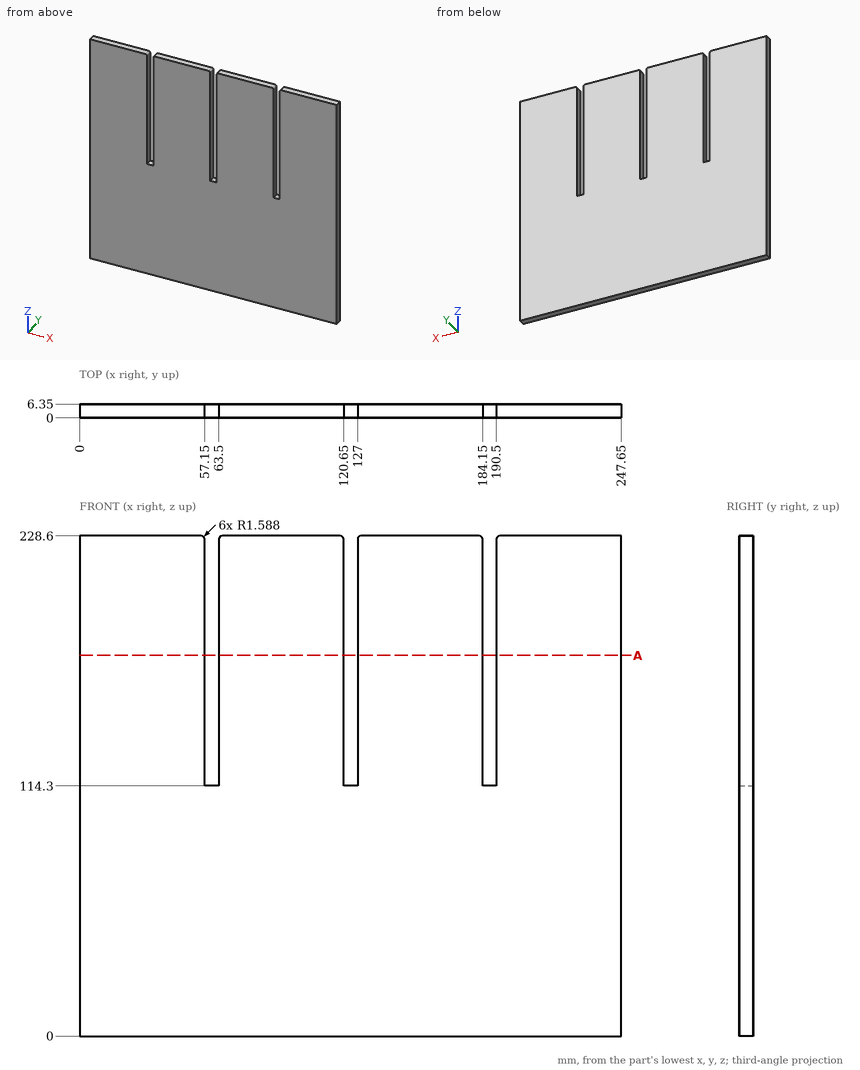
Can you work these out from the drawing? Everything is in mm from the part's minimum corner. Round coordinates to 2 decimals unless told otherwise and drop trailing zeros. Order: outer loops, then holes, each group sorted by start corner. A loop starts at its lowest first (then second) coordinate and runs counter-clockwise, first axis right, second up. Notation, with made-up numbers: (56, 7.5) -> (63, 7.5) arc R19 cw to (63, 27.5) -> close; hole circle Ø6 at (-6.5, 47.25). An arc over 180 degrees is marked (long way). Use CSV: the item, a comma, the result in double quotes.
1. I'm going to push flat-ended pins straight in: P1, Ø1.9, axis at x = 123.5, y = 3.5, coming from the +Z side; P2, Ø3, axis at y = 3, z = 192.5, coming from the -X side. Where does each tip first touch, or does it pass through?
Recorded:
P1,"stops at z = 114.3"
P2,"stops at x = 0"
2. I need wall thicknesses on line 1 along X through (y, z) = (1, 172.5); line 2 along Z through (x, y) = (185.5, 5.5). Which ranges of each line are inside material? Lowest first, please.
Recorded:
line 1,"x = 0 to 57.15, 63.5 to 120.65, 127 to 184.15, 190.5 to 247.65"
line 2,"z = 0 to 114.3"
3. I want a section at A-A on z = 174. List the corners of the cut face in (x, y) for me, and give its area (3 significant figures).
Recorded:
outline,"(0, 0) -> (57.15, 0) -> (57.15, 6.35) -> (0, 6.35) -> close; (63.5, 0) -> (120.65, 0) -> (120.65, 6.35) -> (63.5, 6.35) -> close; (127, 0) -> (184.15, 0) -> (184.15, 6.35) -> (127, 6.35) -> close; (190.5, 0) -> (247.65, 0) -> (247.65, 6.35) -> (190.5, 6.35) -> close"
area,"1,450 mm2"
